```python
from build123d import *

# Parameters (mm, degrees)
SKETCH_1_W          = 50
SKETCH_1_H          = 50
EXTRUDE_1_DEPTH     = 3
SKETCH_2_R          = 7
SKETCH_2_R_2        = 1.6
CUT_EXTRUDE_1_DEPTH = 71.774289117
CUT_EXTRUDE_2_DEPTH = 71.774289117
FILLET_1_R          = 10


with BuildPart() as part:
    # 草图1 → 凸台-拉伸1 (new body)
    with BuildSketch(Plane.XY):
        with Locations((25, -25)):
            Rectangle(SKETCH_1_W, SKETCH_1_H)
    extrude(amount=EXTRUDE_1_DEPTH)

    # 草图2 → 切除-拉伸1 (cut, through all)
    with BuildSketch(Plane.XY.offset(3)):
        with Locations((15, -15)):
            Circle(SKETCH_2_R)
        with Locations((45, -45)):
            Circle(SKETCH_2_R_2)
        with Locations(Location((45, -35, 0), (0, 0, 180))):
            Circle(SKETCH_2_R_2)
        with Locations((25, -35)):
            Circle(SKETCH_2_R_2)
        with Locations(Location((25, -45, 0), (0, 0, 180))):
            Circle(SKETCH_2_R_2)
        with Locations((35, -25)):
            Circle(SKETCH_2_R_2)
    extrude(amount=-CUT_EXTRUDE_1_DEPTH, mode=Mode.SUBTRACT)

    # 草图3 → 切除-拉伸2 (cut, through all)
    with BuildSketch(Plane.XY.offset(3)):
        Polygon((0, -25), (20, -50), (0, -50), align=None)
        Polygon((25, 0), (50, 0), (50, -25), align=None)
    extrude(amount=-CUT_EXTRUDE_2_DEPTH, mode=Mode.SUBTRACT)

    # 圆角1
    fillet_1_edges = [part.edges().sort_by_distance(p)[0] for p in [
        (0, -25, 1.5),
        (20, -50, 1.5),
        (50, -25, 1.5),
        (25, 0, 1.5),
    ]]
    fillet(fillet_1_edges, radius=FILLET_1_R)


solid = part.part
```
CAD build for the part. Positions are in the model's coordinates, mm. Round coordinates to 2 decimals unless told otherwise and drop trailing zeros. Order: outer loops, then holes, each group sorted by start corner. A loop starts at its lowest first (then second) coordinate and runs counter-clockwise, first axis right, second up.
Item 1: Saw through at B-B on x = 15. Write the cut outline in (y, z).
Item 2: Mould opens along X. For faces 1 (the face through (0.55, -24.76, 1.48)), 2 (the face through (24.26, -43.58, 1.52)), 3 (the face through (25, -25, 3)), 4 (the face through (33.82, -23.92, 1.52)) say: pulls with the +X half, pulls with the -X half, needs draft (parallel to the pull), parting line crosses it, or undercut.
Item 3: Saw through at A-A on y = -15. Write the cut outline in (x, z).
Item 4: Saw through at D-D on z = 0.65. Write the cut outline in (x, y).
Item 5: Saw through at C-C on y = -35. Write the cut outline in (x, z).
Item 6: Probe line 1 along X through (y, z) = (-34, 2.65); line 2 along Y through (x, z) = (45, 0.6); line 3 along Y through (x, z) = (25, 0.75). List the from-to ranges inside material, lowest first.
Item 7: Pin check, flat tips, straight feed: pin 1 (3 mm diameter, centred on x = 45, y = -45, fed in from -Z); pin 2 (1.5 mm diameter, centred on x = 29, z = 2, fed in from +Y). Stop position of each tip, or through.
Reported:
1. outline: (-43.75, 0) - (-22, 0) - (-22, 3) - (-43.75, 3) - close; (-8, 0) - (0, 0) - (0, 3) - (-8, 3) - close
2. face 1: pulls with the -X half
2. face 2: undercut
2. face 3: needs draft
2. face 4: undercut
3. outline: (0, 0) - (8, 0) - (8, 3) - (0, 3) - close; (22, 0) - (40, 0) - (40, 3) - (22, 3) - close
4. outline: (0, -21.49) arc R10 ccw to (2.19, -27.74) - (17, -46.25) arc R10 ccw to (24.81, -50) - (50, -50) - (50, -29.14) arc R10 ccw to (47.07, -22.07) - (27.93, -2.93) arc R10 ccw to (20.86, 0) - (0, 0) - close; hole circle Ø14 at (15, -15); hole circle Ø3.2 at (25, -45); hole circle Ø3.2 at (25, -35); hole circle Ø3.2 at (35, -25); hole circle Ø3.2 at (45, -45); hole circle Ø3.2 at (45, -35)
5. outline: (8, 0) - (23.4, 0) - (23.4, 3) - (8, 3) - close; (26.6, 0) - (43.4, 0) - (43.4, 3) - (26.6, 3) - close; (46.6, 0) - (50, 0) - (50, 3) - (46.6, 3) - close
6. line 1: x = 7.2 to 23.75, 26.25 to 43.75, 46.25 to 50
6. line 2: y = -50 to -46.6, -43.4 to -36.6, -33.4 to -20
6. line 3: y = -50 to -46.6, -43.4 to -36.6, -33.4 to -0.9
7. pin 1: passes through
7. pin 2: stops at y = -3.25
